from build123d import *

# Parameters (mm, degrees)
BOSS_EXTRUDE1_DEPTH = 15
SKETCH4_R           = 7.5
CUT_EXTRUDE1_DEPTH  = 128.47548784
SKETCH5_R           = 7.656287761
CUT_EXTRUDE2_DEPTH  = 128.47548784


with BuildPart() as part:
    # Sketch1 → Boss-Extrude1 (new body)
    with BuildSketch(Plane.XY):
        with BuildLine():
            Line((-105, -20), (105, -20))
            ThreePointArc((105, -20), (125, 0), (105, 20))
            Line((105, 20), (-105, 20))
            ThreePointArc((-105, 20), (-125, 0), (-105, -20))
        make_face()
    extrude(amount=BOSS_EXTRUDE1_DEPTH)

    # Sketch4 → Cut-Extrude1 (cut, through all)
    with BuildSketch(Plane.XY.offset(15)):
        with Locations((105, 0)):
            Circle(SKETCH4_R)
    cut_extrude1 = extrude(amount=-CUT_EXTRUDE1_DEPTH, mode=Mode.SUBTRACT)

    # Mirror1: Cut-Extrude1 across plane
    add(cut_extrude1.mirror(Plane(origin=(0, 0, 0), x_dir=(0, 0, 1), z_dir=(1, 0, 0))), mode=Mode.SUBTRACT)

    # Sketch5 → Cut-Extrude2 (cut, through all)
    with BuildSketch(Plane.XY.offset(15)):
        with Locations((55, 0)):
            Circle(SKETCH5_R)
    extrude(amount=-CUT_EXTRUDE2_DEPTH, mode=Mode.SUBTRACT)


solid = part.part
Model file for the job. Use its own axes, mm. Give positions to 0.01 mm unless a question says otherwise; leave off trailing zeros. Order: outer loops, then holes, each group sorted by start corner. A loop starts at its lowest first (then second) coordinate and runs counter-clockwise, first axis right, second up. Notation, with made-up numbers: (81.25, 36) -> (110.25, 36) arc R10 cw to (110.25, 50) -> close; hole circle Ø8 at (14.25, 57.5). An arc over 180 degrees is marked (long way). Use CSV: the item, a comma, the result in double quotes.
1. Drill centre lines: line 1 along Y through (x, z) = (55, 5.25); line 2 along X through (y, z) = (3.5, 10); line 3 along Y through (x, z) = (105, 3.75). Where is each one in solid material? Low to high. Write a range as from..to.
Outcome:
line 1,"-20..-7.66, 7.66..20"
line 2,"-124.69..-111.63, -98.37..48.19, 61.81..98.37, 111.63..124.69"
line 3,"-20..-7.5, 7.5..20"
2. Band-saw the part on A-A, the plane z = 8.5. Give the cut face in (x, y), then the cut area to 3 significant figures.
Outcome:
outline,"(-105, -20) -> (105, -20) arc R20 ccw to (105, 20) -> (-105, 20) arc R20 ccw to start; hole circle Ø15 at (-105, 0); hole circle Ø15.31 at (55, 0); hole circle Ø15 at (105, 0)"
area,"9,120 mm²"
3. Mould opens along Y. For faces 1 (the cylindrical face through (125, 0, 7)), 2 (the cylindrical face through (112.154, 2.253, 7.605)), 3 (the flat face through (-2, 0, 15)) say: +Y half, -Y half, draft (parallel to the pull), parting line (faces both ways), or undercut.
Outcome:
face 1,"parting line"
face 2,"undercut"
face 3,"draft"
4. Band-saw the part on B-B, the plane x = 55. Give the cut face in (y, z).
Outcome:
outline,"(-20, 0) -> (-7.66, 0) -> (-7.66, 15) -> (-20, 15) -> close; (7.66, 0) -> (20, 0) -> (20, 15) -> (7.66, 15) -> close"
5. Band-saw the part on D-D, the plane y = 12. Give the cut face in (x, z).
Outcome:
outline,"(-121, 0) -> (121, 0) -> (121, 15) -> (-121, 15) -> close"
6. Band-saw the part on C-C, the plane y = 0. Give the cut face in (x, z), then the cut area to 3 significant figures.
Outcome:
outline,"(-125, 0) -> (-112.5, 0) -> (-112.5, 15) -> (-125, 15) -> close; (-97.5, 0) -> (47.34, 0) -> (47.34, 15) -> (-97.5, 15) -> close; (62.66, 0) -> (97.5, 0) -> (97.5, 15) -> (62.66, 15) -> close; (112.5, 0) -> (125, 0) -> (125, 15) -> (112.5, 15) -> close"
area,"3,070 mm²"
